Geometry: final body of the model. Coordinates: model frame, mm. Face numbers are marked on the shaded views. A direction names the side the tool comes from. Give positions to 0.01 mm unless a question says otherwise; leave off trailing zeros. Write each loop counter-clockwise with the first axis right and the second up, starting at its lowest first coordinate (ties: lowest second). Pieces come first, ordered by that corner, then holes.
Q1. Draft query along Y for the marked faces 1 and 2. Return one class per face: pulls with the +Y half, pulls with the -Y half, needs draft (parallel to the pull), parting line crosses it, or undercut.
Q2. Reachability of the marked faces 3 and 4 from +Z, -Z, +X, -X, +Y, -Y: full face, straight path, thin tool, end or side. Return the list, or none.
Q3. Cut plane A-A on y = 0. Return the cut outline in (x, z) (3 decimals), plus the area to 4 significant figures.
Q4. Cut plane C-C on z = -1.3. Return the cut outline in (x, y), plus the area to 3 significant figures.
Q5. Line query: L1, parallel to Y at x = 0, z = -0.45; L2, parallel to X at y = -6.5, z = -0.7; L3, parallel to Y at x = 1.25, z = -0.75. Output: solid intervals per line, ascending.
Autodesk Inventor part; units mm, degrees
ref_plane "YZ Plane" through (0, 0, 0) normal (1, 0, 0) x (0, 1, 0)
ref_plane "XZ Plane" through (0, 0, 0) normal (0, 1, 0) x (-1, 0, 0)
ref_plane "XY Plane" through (0, 0, 0) normal (0, 0, 1) x (1, 0, 0)
sketch "Sketch1" plane through (0, 0, 0) normal (0, 0, 1) x (1, 0, 0)
  circle A0 centre (0, 0) radius 10
  circle A1 centre (0, 0) radius 13.5
  circle A2 centre (0, 0) radius 12.5
  circle A3 centre (0, 0) radius 11
  dimension "d0" = 20
  dimension "d1" = 27
  dimension "d2" = 1
  dimension "d3" = 1
extrude "Extrusion1" add sketch "Sketch1" along normal mid plane 4
extrude "Extrusion2" add sketch "Sketch1" along normal mid plane 3.75 contours A2
properties part number "6704ZZ" material "Steel, Carbon"
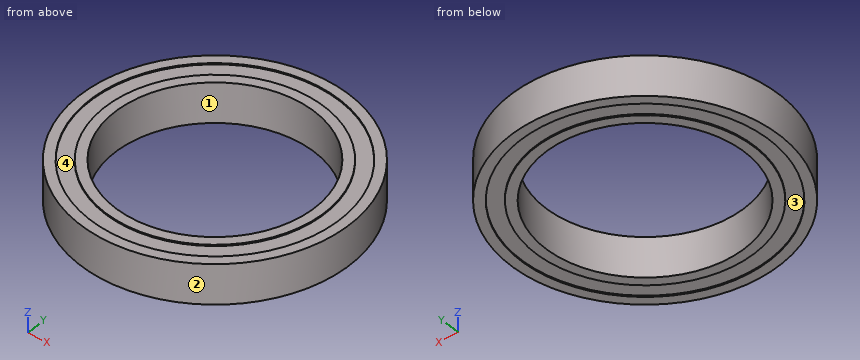
Data:
1. face 1: undercut
1. face 2: parting line crosses it
2. face 3: -Z
2. face 4: +Z
3. outline: (-13.5, -2) - (-12.5, -2) - (-12.5, -1.875) - (-11, -1.875) - (-11, -2) - (-10, -2) - (-10, 2) - (-11, 2) - (-11, 1.875) - (-12.5, 1.875) - (-12.5, 2) - (-13.5, 2) - close; (10, -2) - (11, -2) - (11, -1.875) - (12.5, -1.875) - (12.5, -2) - (13.5, -2) - (13.5, 2) - (12.5, 2) - (12.5, 1.875) - (11, 1.875) - (11, 2) - (10, 2) - close
3. area: 27.25 mm2
4. outline: circle Ø27 at (0, 0); hole circle Ø20 at (0, 0)
4. area: 258 mm2
5. L1: y = -13.5 to -10, 10 to 13.5
5. L2: x = -11.83 to -7.6, 7.6 to 11.83
5. L3: y = -13.44 to -9.92, 9.92 to 13.44
